Build history of the part. All positions in model axes, mm. A direction names the side the tool comes from. Give positions to 0.01 mm unless a question says otherwise; leave off trailing zeros. Order: outer loops, then holes, each group sorted by start corner. A loop starts at its lowest first (then second) coordinate and runs counter-clockwise, first axis right, second up. Notation, with made-up numbers: M -36.75,15.25 L -22.75,15.25 A26 cw -22.75,52.25 Z; hole C 36,25 d6. An arc over 180 degrees is marked long. Answer as CSV lines item,"result".
from build123d import *

# Parameters (mm, degrees)
SKETCH1_W               = 50.8
SKETCH1_H               = 50.8
SKETCH1_R               = 13.49375
BOSS_EXTRUDE1_DEPTH     = 6.35
LPATTERN2_COUNT         = 2
LPATTERN2_PITCH         = 9.398
SKETCH2_W               = 50.8
SKETCH2_H               = 50.8
SKETCH2_R               = 11.90625
BOSS_EXTRUDE2_DEPTH     = 1.190625
SKETCH3_R               = 1.82499
CUT_EXTRUDE1_DEPTH      = 19.05
SKETCH5_R               = 15.875
CUT_EXTRUDE2_DEPTH      = 6.35
CUT_EXTRUDE3_REACH      = 60.939
CUT_EXTRUDE3_END_RADIUS = 15.875
SKETCH6_R               = 1.82499
SKETCH7_R               = 6.35
BOSS_EXTRUDE3_DEPTH     = 15.24
SKETCH8_R               = 3.175
BOSS_EXTRUDE4_DEPTH     = 9.398


with BuildPart() as part:
    # Sketch1 → Boss-Extrude1 (new body)
    with BuildSketch(Plane.XY):
        Rectangle(SKETCH1_W, SKETCH1_H)
        Circle(SKETCH1_R, mode=Mode.SUBTRACT)
    extrude(amount=BOSS_EXTRUDE1_DEPTH)


with BuildPart() as lpattern2_1:
    # LPattern2: pattern copy
    add(part.part.moved(Location(Vector(0, 0, 1) * (1 * LPATTERN2_PITCH))))

    # Sketch5 → Cut-Extrude2 (cut)
    with BuildSketch(Plane.XY.offset(15.748)):
        Circle(SKETCH5_R)
    extrude(amount=-CUT_EXTRUDE2_DEPTH, mode=Mode.SUBTRACT)

    # Cut-Extrude3: up to this cylinder (the profile starts outside it)
    cut_extrude3_end = Plane(origin=(0, 0, 12.573), z_dir=(0, 0, 1)) * Cylinder(CUT_EXTRUDE3_END_RADIUS, 154.628, mode=Mode.PRIVATE)
    # Sketch6 → Cut-Extrude3 (cut, up to the surface)
    with BuildSketch(Plane.XZ.offset(25.4), mode=Mode.PRIVATE) as cut_extrude3_sk1:
        with Locations(Location((0, 12.573, 0), (0, 0, 270))):
            Circle(SKETCH6_R)
    cut_extrude3_tool1 = extrude(cut_extrude3_sk1.sketch, amount=-CUT_EXTRUDE3_REACH, mode=Mode.PRIVATE) - cut_extrude3_end
    add(cut_extrude3_tool1.solids().sort_by_distance((0, -25.4, 12.573))[0], mode=Mode.SUBTRACT)

    # Sketch7 → Boss-Extrude3 (add)
    with BuildSketch(Plane.XY.offset(15.748)):
        with Locations((19.05, -19.05)):
            Circle(SKETCH7_R)
        with Locations(Location((-19.05, 19.05, 0), (0, 0, 180))):
            Circle(SKETCH7_R)
    extrude(amount=BOSS_EXTRUDE3_DEPTH)


with BuildPart() as part_1:
    add(part.part)

    # Sketch2 → Boss-Extrude2 (add)
    with BuildSketch(Plane.XY.offset(6.35)):
        Rectangle(SKETCH2_W, SKETCH2_H)
        Circle(SKETCH2_R, mode=Mode.SUBTRACT)
    extrude(amount=-BOSS_EXTRUDE2_DEPTH)

    # Sketch3 → Cut-Extrude1 (cut)
    with BuildSketch(Plane(origin=(0, 25.4, 0), x_dir=(1, 0, 0), z_dir=(0, 1, 0))):
        with Locations(Location((0, -3.175, 0), (0, 0, 270))):
            Circle(SKETCH3_R)
    extrude(amount=-CUT_EXTRUDE1_DEPTH, mode=Mode.SUBTRACT)

    add(lpattern2_1.part)  # Boss-Extrude4 merges LPattern2_1
    # Sketch8 → Boss-Extrude4 (add)
    with BuildSketch(Plane(origin=(0, 0, 9.398), x_dir=(-1, 0, 0), z_dir=(0, 0, -1))):
        with Locations((-19.05, -19.05)):
            Circle(SKETCH8_R)
        with Locations((19.05, 19.05)):
            Circle(SKETCH8_R)
    extrude(amount=BOSS_EXTRUDE4_DEPTH)


solid = part_1.part
Item 1: Band-saw the part on D-D (z = 12). Give the cut face in (x, y) (3 decimals).
Geometry says:
outline,"M -25.4,-25.4 L -1.733,-25.4 L -1.733,-15.78 A15.875 cw long 1.733,-15.78 L 1.733,-25.4 L 25.4,-25.4 L 25.4,25.4 L -25.4,25.4 Z"
Item 2: 3-axis set-ups, long thin cutter, end or side, ignore diameter. For faces 1 (the flat face through (24, -24, 15.748)), 2 (the cylindrical face through (-0.7, 19.47, 4.86)), 3 (the cylindrical face through (24.916, -21.482, 23.261)), 4 (the flat face through (-24, 24, 15.748)), 5 (the cylindrical face through (0.08, -20.652, 14.396)): which of +Z, -Z, +X, -X, +Y, -Y reach the whole face in a straight line?
Geometry says:
face 1,"+Z, +X, -Y"
face 2,"+Y"
face 3,"+Z"
face 4,"+Z, -X, +Y"
face 5,"-Y"
Item 3: Band-saw the part on A-A (y = 0). Give the cut face in (x, z) (3 decimals).
Geometry says:
outline,"M -25.4,0 L -13.494,0 L -13.494,5.159 L -11.906,5.159 L -11.906,6.35 L -25.4,6.35 Z; M -25.4,9.398 L -15.875,9.398 L -15.875,15.748 L -25.4,15.748 Z; M 11.906,5.159 L 13.494,5.159 L 13.494,0 L 25.4,0 L 25.4,6.35 L 11.906,6.35 Z; M 15.875,9.398 L 25.4,9.398 L 25.4,15.748 L 15.875,15.748 Z"
Item 4: Band-saw the part on C-C (y = -20.5). Give the cut face in (x, z).
Geometry says:
outline,"M -25.4,0 L 25.4,0 L 25.4,6.35 L 21.87,6.35 L 21.87,9.4 L 25.4,9.4 L 25.4,15.75 L 25.23,15.75 L 25.23,30.99 L 12.87,30.99 L 12.87,15.75 L -25.4,15.75 L -25.4,9.4 L 16.23,9.4 L 16.23,6.35 L -25.4,6.35 Z; hole C 0,12.57 d3.65"
Item 5: Band-saw the part on B-B (z = 19.5). Give the cut face in (x, y), and give its area (3 significant figures).
Geometry says:
outline,"C -19.05,19.05 d12.7; C 19.05,-19.05 d12.7"
area,"253 mm2"
Item 6: Probe line 1 along Z through (x, y) = (0, -18); line 2 along X through (y, z) = (0, 2); line 3 along Z through (x, y) = (2, -23). List the from-to ranges inside material, lowest first. Write a range as from..to.
Geometry says:
line 1,"z = 0..6.35, 9.4..10.75, 14.4..15.75"
line 2,"x = -25.4..-13.49, 13.49..25.4"
line 3,"z = 0..6.35, 9.4..15.75"
Item 7: Pull direction X, two halves, no side cores. Call faces 6 (the flat face through (11, 12, 9.398)), 7 (the cylindrical face through (-2.93, -13.17, 2.54)), 8 (the flat face through (25.4, 0, 3)): released by +X, released by -X, zero draft, split by the parting line, or undercut.
Geometry says:
face 6,"zero draft"
face 7,"undercut"
face 8,"released by +X"
Item 8: Drop flat-ended pins along their axis: pin 1 (4 mm diameter, centred on x = 12.5, y = 15.5, fed in from -Z); pin 2 (1 mm diameter, centred on x = -14, z = 17.5, fed in from +Y); pin 3 (5 mm diameter, centred on x = 15.5, y = 17.5, fed in from +Z). Give the stop position or say it passes through.
Geometry says:
pin 1,"stops at z = 0"
pin 2,"stops at y = 23.48"
pin 3,"stops at z = 15.75"
